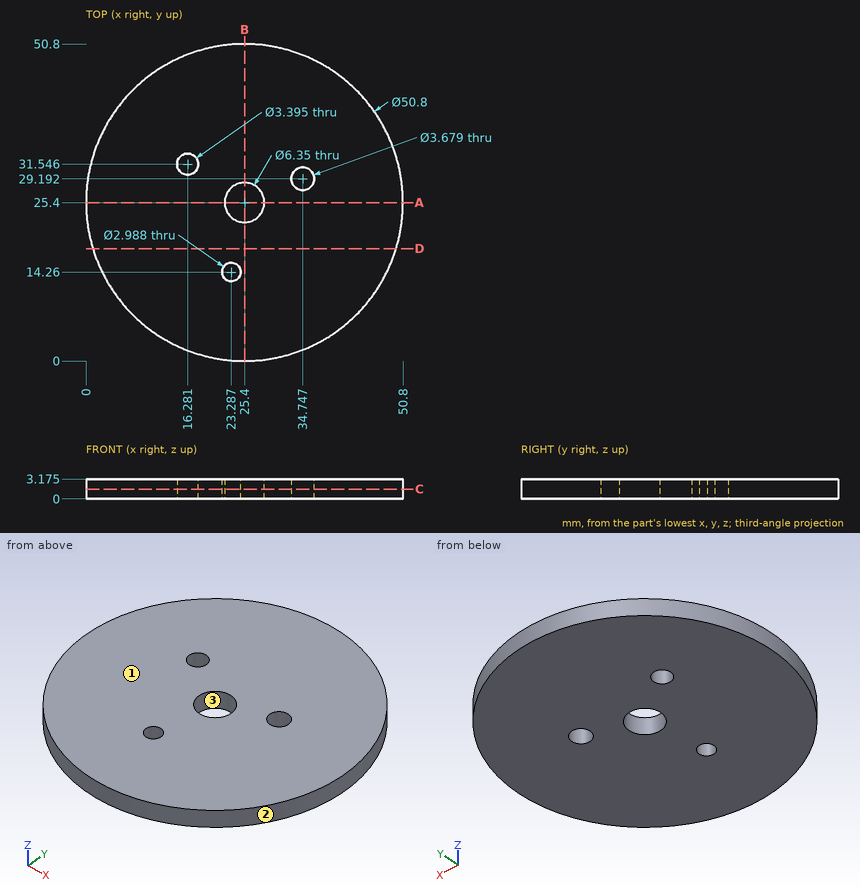
The figure shows three views and two pictorial views of one solid part (mm, origin at its lowest corner). Answer the questions. Coordinates: 2 decimals unless noted, no trailing zeros. Loops run counter-clockwise (first coordinate to the right, second up) from the corner with the lowest first, then second, coordinate; pieces in that order, holes last. Notation, with made-up numbers: M -40,-31.75 L -13,-31.75 A21 cw -13,-27.75 Z; hole C -26.5,28.25 d6. An arc over 180 degrees is marked long. Answer as CSV lines item,"result". Start each with the question number.
(1) The part is cut by section A-A (y = 25.4). Give the vertices of the cut face in (x, z) (1 decimal), and give its area (3 significant figures).
(2) Given pin 1 (1 mm diameter, centred on x = 32.5, z = 2, fed in from -Y), flat-ended and moving along its own axis, determine where the tip first touches the part or whether it passes through.
(3) The part is cut by section D-D (y = 18). Give the vertices of the cut face in (x, z) (1 decimal), and give its area (3 significant figures).
(4) Find the intervals of material crossed by L1, parallel to Y at x = 25.4, z = 0.75 (1 decimal); L2, parallel to Y at x = 36, z = 2.7 (1 decimal); L3, parallel to Y at x = 23, z = 2.5 (1 decimal), in increasing order. Write a range as [from, to].
(5) The mould has two halves that part along X. Classify the marked faces 1, 2 and 3: pulls with the +X half, pulls with the -X half, needs draft (parallel to the pull), parting line crosses it, or undercut.
(6) The part is cut by section C-C (z = 1.55). State how many separate pieces and enclosed holes the cut face has, and give its area (3 significant figures).
Determined:
1,outline,"M 0,0 L 22.2,0 L 22.2,3.2 L 0,3.2 Z; M 28.6,0 L 50.8,0 L 50.8,3.2 L 28.6,3.2 Z"
1,area,"141 mm2"
2,pin 1,"y = 0.87"
3,outline,"M 1.1,0 L 49.7,0 L 49.7,3.2 L 1.1,3.2 Z"
3,area,"154 mm2"
4,L1,"[0, 22.2], [28.6, 50.8]"
4,L2,"[2.3, 27.8], [30.5, 48.5]"
4,L3,"[0.1, 12.8], [15.7, 23.3], [27.5, 50.7]"
5,face 1,"needs draft"
5,face 2,"parting line crosses it"
5,face 3,"undercut"
6,separate pieces,"1"
6,enclosed holes,"4"
6,area,"1,970 mm2"
